The model under review builds one solid part; all positions refer to its coordinate system, in mm. Coordinates: 2 decimals unless noted, no trailing zeros. Order: outer loops, then holes, each group sorted by start corner. A loop starts at its lowest first (then second) coordinate and runs counter-clockwise, first axis right, second up. Notation, with made-up numbers: M 14,-7.75 L 25,-7.75 A6 cw 25,-0.75 Z; hole C -14.75,85 d10. An arc over 180 degrees is marked long. Answer as CSV lines item,"result". Start each with the question number.
Q1. Consider section A-A on z = 4.1. Write out the cut boundary in (x, y), and give its area (3 significant figures).
Q2. Wall thickness on L1, parallel to X at y = 0, z = 3.5; L2, parallel to X at y = 6, z = 4.95: over which ranges is each line inside the solid? List them lowest first. Write a range as [from, to].
Q3. Consider section B-B on x = 0. Write out the cut boundary in (y, z) (3 decimals).
Q4. The part is to be moulded in two halves that separate along Y. For faces 1 (the face through (2.44, 0.54, 2.78)), 2 (the face through (-6.665, 6.649, 2.788)), 3 (the face through (-6.95, 0, 3)), say which applies: +Y half, -Y half, draft (parallel to the pull), parting line (faces both ways), or undercut.
from build123d import *

# Parameters (mm, degrees)
SKETCH_1_W      = 13.9
SKETCH_1_H      = 13.9
EXTRUDE_1_DEPTH = 5.5
FILLET_1_R      = 1


with BuildPart() as part:
    # Эскиз1 → Бобышка-Вытянуть1 (new body)
    with BuildSketch(Plane.XY):
        Rectangle(SKETCH_1_W, SKETCH_1_H)
    extrude(amount=EXTRUDE_1_DEPTH)

    # Эскиз3 → Отверстие обработанное метчиком M61 (revolve, cut)
    with BuildSketch(Plane(origin=(0, 0, 5.5), x_dir=(0, -1, 0), z_dir=(1, 0, 0))):
        Polygon((0, 0), (0, 5.5), (3.025, 5.5), (2.5, 4.975), (2.5, 0.525), (3.025, 0), align=None)
    revolve(axis=Axis((0, 0, 11.85), (0, 0, -1)), mode=Mode.SUBTRACT)

    # Скругление1
    fillet_1_edges = [part.edges().sort_by_distance(p)[0] for p in [
        (6.95, -6.95, 2.75),
        (-6.95, -6.95, 2.75),
        (-6.95, 6.95, 2.75),
        (6.95, 6.95, 2.75),
    ]]
    fillet(fillet_1_edges, radius=FILLET_1_R)


solid = part.part
Evaluation:
1,outline,"M -6.95,-5.95 A1 ccw -5.95,-6.95 L 5.95,-6.95 A1 ccw 6.95,-5.95 L 6.95,5.95 A1 ccw 5.95,6.95 L -5.95,6.95 A1 ccw -6.95,5.95 Z; hole C 0,0 d5"
1,area,"173 mm²"
2,L1,"x = [-6.95, -2.5], [2.5, 6.95]"
2,L2,"x = [-6.95, 6.95]"
3,outline,"M -6.95,0 L -3.025,0 L -2.5,0.525 L -2.5,4.975 L -3.025,5.5 L -6.95,5.5 Z; M 2.5,0.525 L 3.025,0 L 6.95,0 L 6.95,5.5 L 3.025,5.5 L 2.5,4.975 Z"
4,face 1,"undercut"
4,face 2,"+Y half"
4,face 3,"draft"
